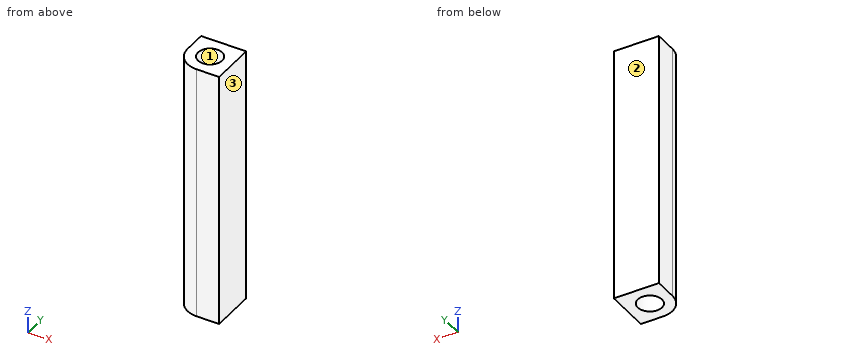
```python
from build123d import *

# Parameters (mm, degrees)
F0_W      = 14
F0_H      = 14
F0_R      = 3.75
F1_DEPTH  = 70
F1_FACE_W = 14
F1_FACE_H = 14
F1_FACE_R = 3.75
F2_DEPTH  = 10
F3_R      = 7


with BuildPart() as f1:
    # F0 (on Top) → F1 (new body)
    with BuildSketch(Plane.XY):
        Rectangle(F0_W, F0_H)
        Circle(F0_R, mode=Mode.SUBTRACT)
    extrude(amount=F1_DEPTH)

    # F1_face (on face) → F2 (join)
    with BuildSketch(Plane.XY.offset(70)):
        Rectangle(F1_FACE_W, F1_FACE_H)
        Circle(F1_FACE_R, mode=Mode.SUBTRACT)
    extrude(amount=F2_DEPTH)

    # F3
    f3_edges = [f1.edges().sort_by_distance(p)[0] for p in [
        (-7, -7, 40),
    ]]
    fillet(f3_edges, radius=F3_R)


solid = f1.part
```
CAD build for the part. Positions are in the model's coordinates, mm. Face numbers are marked on the shaded views. Round coordinates to 2 decimals unless told otherwise and drop trailing zeros. Loops run counter-clockwise (first coordinate to the right, second up) from the corner with the lowest first, then second, coordinate; pieces in that order, holes last. Notation, with made-up numbers: M 62.25,-18.5 L 67.25,-18.5 A16 cw 67.25,12.5 Z; hole C 71.5,84.5 d11. An arc over 180 degrees is marked long. Use a Markdown table: item, result. Add a question column.
(1) Cut at C-C (x = 0.75). Give the cut face in (y, z).
(2) Drill centre lines: line 1 (Y direction, x = 0, z = 42.5); line 2 (Y direction, x = -2, z = 35); line 3 (X direction, y = 0.75, z = 39). Where is each one in solid material? Low to high.
(3) Flat gauge pin, fed straight in: pin 1 (2 mm diameter, centred on x = -5.5, z = 26, fed in from -Y). Where does the tip first touch, or does it go through?
(4) Cut at A-A (y = 2.25). Give the cut face in (x, z), and give its area (3 significant figures).
(5) Cut at D-D (y = -4.5). Give the cut face in (x, z), and give its area (3 significant figures).
(6) Cut at B-B (z = 44). Give the cut face in (x, y), and give its area (3 significant figures).
(7) Pull direction X, two halves, no side cores. Call the marked faces 1, 2 and 3: +X half, -X half, draft (parallel to the pull), parting line (faces both ways), or undercut.
Geometry says:
| question | item | result |
|---|---|---|
| 1 | outline | M -7,0 L -3.67,0 L -3.67,80 L -7,80 Z; M 3.67,0 L 7,0 L 7,80 L 3.67,80 Z |
| 2 | line 1 | y = -7 to -3.75, 3.75 to 7 |
| 2 | line 2 | y = -6.71 to -3.17, 3.17 to 7 |
| 2 | line 3 | x = -7 to -3.67, 3.67 to 7 |
| 3 | pin 1 | stops at y = -5.36 |
| 4 | outline | M -7,0 L -3,0 L -3,80 L -7,80 Z; M 3,0 L 7,0 L 7,80 L 3,80 Z |
| 4 | area | 640 mm² |
| 5 | outline | M -5.36,0 L 7,0 L 7,80 L -5.36,80 Z |
| 5 | area | 989 mm² |
| 6 | outline | M -7,0 A7 ccw 0,-7 L 7,-7 L 7,7 L -7,7 Z; hole C 0,0 d7.5 |
| 6 | area | 141 mm² |
| 7 | face 1 | undercut |
| 7 | face 2 | draft |
| 7 | face 3 | +X half |
